Input: part model. Units: mm. Frame: model coordinates. Face numbers are marked on the shaded views. A direction names the side the tool comes from. Round coordinates to 2 decimals unless told otherwise and drop trailing zeros. Loops run counter-clockwise (first coordinate to the right, second up) from the corner with the lowest first, then second, coordinate; pieces in that order, holes last. Notation, with made-up numbers: (37, 5.25) - (81, 5.25) arc R13 ccw to (81, 28.25) - close; hole circle Ø3 at (43, 29). An arc over 180 degrees is marked (long way). One line per question, with ' | ' between items. Start each with the question number.
Item 1: Section C-C, the plane x = 14.5. Return loops of the section in (y, z), plus the area to 3 significant figures.
Item 2: Section A-A, the plane y = 0. Give the number of separate pieces and of enclosed holes in the cut face, plus the area to 3 significant figures.
Item 3: Set-up query: the marked faces 5, 6 and 7. Return all of +Z, -Z, +X, -X, +Y, -Y with unobstructed straight access to the full face (end or side cutting, diameter ignored); none if empty.
Item 4: First-contact query: pin 1 (6.5 mm diameter, centred on x = 8.5, y = 8, fed in from -Z); pin 2 (2 mm diameter, centred on y = -17.5, z = 0.5, fed in from +X); pin 3 (1.8 mm diameter, centred on x = -14.5, z = 3.5, fed in from +Y). Flat tips, straight axial feed; report the tip coordinate or a pass-through.
Item 5: Section D-D, the plane z = 3.25. Return loops of the section in (x, y), plus the area to 3 significant figures.
Item 6: Material intervals for line 1 along Y through (x, z) = (3.5, 1.25); line 2 along X through (y, z) = (0, 1.55); line 3 along Y through (x, z) = (-8, 1), sorted ascending.
Item 7: Draft query along X for the marked faces 1, 2, 3 and 4. Return one class per face: pulls with the +X half, pulls with the -X half, needs draft (parallel to the pull), parting line crosses it, or undercut.
```python
from build123d import *

# Parameters (mm, degrees)
SKETCH_1_R               = 17.4
EXTRUDE_1_DEPTH          = 5.6
SKETCH_2_R               = 1.7
CUT_EXTRUDE_1_DEPTH      = 26.23648153
SKETCH_3_R               = 7
CUT_EXTRUDE_2_DEPTH      = 26.23648153
SKETCH_4_R               = 2.8
CUT_EXTRUDE_3_DEPTH      = 3
SKETCH_5_R               = 1.7
CUT_EXTRUDE_4_DEPTH      = 26.23648153
CUT_EXTRUDE_5_DEPTH      = 2.5
SKETCH_7_W               = 16.1
SKETCH_7_H               = 16.1
CUT_EXTRUDE_6_DEPTH      = 1.5
CHAMFER_1_SIZE           = 0.5
SKETCH_9_W               = 2.2
SKETCH_9_H               = 8
SKETCH_9_W_2             = 8
SKETCH_9_H_2             = 2.2
CUT_EXTRUDE_7_DEPTH      = 26.281613873
BOSS_EXTRUDE1_DEPTH      = 5.6
BOSS_EXTRUDE1_DEPTH_BACK = 4
SKETCH1_R                = 20.65
SKETCH1_R_2              = 17.4
SKETCH3_R                = 23
SKETCH3_R_2              = 20.65
BOSS_EXTRUDE2_DEPTH      = 2.5
SKETCH4_R                = 18
CUT_EXTRUDE3_DEPTH       = 4
SKETCH5_W                = 1
SKETCH5_H                = 8
CUT_EXTRUDE4_DEPTH       = 10
CUT_EXTRUDE6_DEPTH       = 10
FILLET3_R                = 1


with BuildPart() as part:
    # 草图1 → 凸台-拉伸1 (new body)
    with BuildSketch(Plane.XY):
        Circle(SKETCH_1_R)
    extrude(amount=EXTRUDE_1_DEPTH)

    # 草图2 → 切除-拉伸1 (cut, through all)
    with BuildSketch(Plane.XY.offset(5.6)):
        with Locations((-6.717514421, 6.717514421)):
            Circle(SKETCH_2_R)
        with Locations((6.717514421, -6.717514421)):
            Circle(SKETCH_2_R)
    extrude(amount=-CUT_EXTRUDE_1_DEPTH, mode=Mode.SUBTRACT)

    # 草图3 → 切除-拉伸2 (cut, through all)
    with BuildSketch(Plane.XY.offset(5.6)):
        Circle(SKETCH_3_R)
    extrude(amount=-CUT_EXTRUDE_2_DEPTH, mode=Mode.SUBTRACT)

    # 草图4 → 切除-拉伸3 (cut)
    with BuildSketch(Plane.XY.offset(5.6)):
        with Locations((-6.717514421, 6.717514421)):
            Circle(SKETCH_4_R)
        with Locations((6.717514421, -6.717514421)):
            Circle(SKETCH_4_R)
    extrude(amount=-CUT_EXTRUDE_3_DEPTH, mode=Mode.SUBTRACT)

    # 草图5 → 切除-拉伸4 (cut, through all)
    with BuildSketch(Plane.XY.offset(5.6)):
        with Locations((8.05, 8)):
            Circle(SKETCH_5_R)
        with Locations((-8.05, -8)):
            Circle(SKETCH_5_R)
    extrude(amount=-CUT_EXTRUDE_4_DEPTH, mode=Mode.SUBTRACT)

    # 草图6 → 切除-拉伸5 (cut)
    with BuildSketch(Plane(origin=(0, 0, 0), x_dir=(-1, 0, 0), z_dir=(0, 0, -1))):
        Polygon((4.766838493, -8), (6.408419246, -10.84330127), (9.691580754, -10.84330127), (11.333161507, -8), (9.691580754, -5.15669873), (6.408419246, -5.15669873), align=None)
        Polygon((-4.766838493, 8), (-6.408419246, 10.84330127), (-9.691580754, 10.84330127), (-11.333161507, 8), (-9.691580754, 5.15669873), (-6.408419246, 5.15669873), align=None)
    extrude(amount=-CUT_EXTRUDE_5_DEPTH, mode=Mode.SUBTRACT)

    # 草图7 → 切除-拉伸6 (cut)
    with BuildSketch(Plane.XY.offset(5.6)):
        Rectangle(SKETCH_7_W, SKETCH_7_H)
    extrude(amount=-CUT_EXTRUDE_6_DEPTH, mode=Mode.SUBTRACT)

    # 倒角1
    chamfer_1_edges = [part.edges().sort_by_distance(p)[0] for p in [
        (8.05, 1.022551258, 5.6),
        (1.047918985, 8.05, 5.6),
        (-8.05, -1.022551258, 5.6),
        (-1.047918985, -8.05, 5.6),
    ]]
    chamfer(chamfer_1_edges, length=CHAMFER_1_SIZE)

    # 草图8 → 旋转1 (revolve)
    with BuildSketch(Plane(origin=(0, 0, 0), x_dir=(0, 0, -1), z_dir=(1, 0, 0)), mode=Mode.PRIVATE) as revolve_1_sk:
        Polygon((0, 17.4), (0, 17.2), (0.2, 17.4), align=None)
    revolve(revolve_1_sk.sketch.rotate(Axis((0, 0, 0), (0, 0, 1)), 90), axis=Axis((0, 0, 0), (0, 0, 1)))

    # 草图9 → 切除-拉伸7 (cut, through all)
    with BuildSketch(Plane.XY.offset(5.6)):
        with Locations((14.6, 0)):
            Rectangle(SKETCH_9_W, SKETCH_9_H)
        with Locations((0, 14.6)):
            Rectangle(SKETCH_9_W_2, SKETCH_9_H_2)
        with Locations((-14.6, 0)):
            Rectangle(SKETCH_9_W, SKETCH_9_H)
        with Locations((0, -14.6)):
            Rectangle(SKETCH_9_W_2, SKETCH_9_H_2)
    extrude(amount=-CUT_EXTRUDE_7_DEPTH, mode=Mode.SUBTRACT)

    # Sketch1 → Boss-Extrude1 (add, two sides: drawn at the far end of the back side and taken through both)
    with BuildSketch(Plane.XY.offset(-BOSS_EXTRUDE1_DEPTH_BACK)):
        Circle(SKETCH1_R)
        Circle(SKETCH1_R_2, mode=Mode.SUBTRACT)
    extrude(amount=BOSS_EXTRUDE1_DEPTH + BOSS_EXTRUDE1_DEPTH_BACK)

    # Sketch3 → Boss-Extrude2 (add)
    with BuildSketch(Plane(origin=(0, 0, -4), x_dir=(-1, 0, 0), z_dir=(0, 0, -1))):
        Circle(SKETCH3_R)
        with Locations(Location((0, 0, 0), (0, 0, 180))):
            Circle(SKETCH3_R_2, mode=Mode.SUBTRACT)
    extrude(amount=-BOSS_EXTRUDE2_DEPTH)

    # Sketch4 → Cut-Extrude3 (cut)
    with BuildSketch(Plane(origin=(0, 0, -4), x_dir=(-1, 0, 0), z_dir=(0, 0, -1))):
        Circle(SKETCH4_R)
    extrude(amount=-CUT_EXTRUDE3_DEPTH, mode=Mode.SUBTRACT)

    # Sketch5 → Cut-Extrude4 (cut)
    with BuildSketch(Plane(origin=(0, 0, -4), x_dir=(-1, 0, 0), z_dir=(0, 0, -1))):
        with Locations((22.5, 0)):
            Rectangle(SKETCH5_W, SKETCH5_H)
        with Locations((-22.5, 0)):
            Rectangle(SKETCH5_W, SKETCH5_H)
    extrude(amount=-CUT_EXTRUDE4_DEPTH, mode=Mode.SUBTRACT)

    # Sketch7 → Cut-Extrude6 (cut)
    with BuildSketch(Plane(origin=(0, 0, -4), x_dir=(-1, 0, 0), z_dir=(0, 0, -1))):
        with BuildLine():
            Line((0, 18), (0, 22.3))
            Line((0, 22.3), (-2.6, 22.3))
            Line((-2.6, 22.3), (-2.6, 17.811232411))
            ThreePointArc((-2.6, 17.811232411), (-1.303421766, 17.952746077), (0, 18))
        make_face()
        with BuildLine():
            Line((0, 17.5), (0, 18))
            ThreePointArc((0, 18), (-1.303421766, 17.952746077), (-2.6, 17.811232411))
            Line((-2.6, 17.811232411), (-2.6, 17.5))
            Line((-2.6, 17.5), (0, 17.5))
        make_face()
        with BuildLine():
            Line((2.6, 22.3), (0, 22.3))
            Line((0, 22.3), (0, 18))
            ThreePointArc((0, 18), (1.303421766, 17.952746077), (2.6, 17.811232411))
            Line((2.6, 17.811232411), (2.6, 22.3))
        make_face()
        with BuildLine():
            ThreePointArc((2.6, 17.811232411), (1.303421766, 17.952746077), (0, 18))
            Line((0, 18), (0, 17.5))
            Line((0, 17.5), (2.6, 17.5))
            Line((2.6, 17.5), (2.6, 17.811232411))
        make_face()
    extrude(amount=-CUT_EXTRUDE6_DEPTH, mode=Mode.SUBTRACT)

    # Fillet3
    # the kernel refuses this fillet: 1 mm, written as the material it adds along each edge
    with BuildSketch(Plane(origin=(2.6, 22.3, -4), x_dir=(-1, 0, 0), z_dir=(0, 0, 1))) as fillet3_piece_1:
        with BuildLine():
            CenterArc((FILLET3_R, FILLET3_R), FILLET3_R, 180, 90)
            Line((0, FILLET3_R), (-FILLET3_R * 0.02, FILLET3_R))
            Line((-FILLET3_R * 0.02, FILLET3_R), (-FILLET3_R * 0.02, -FILLET3_R * 0.02))
            Line((-FILLET3_R * 0.02, -FILLET3_R * 0.02), (FILLET3_R, -FILLET3_R * 0.02))
            Line((FILLET3_R, -FILLET3_R * 0.02), (FILLET3_R, 0))
        make_face()
    extrude(amount=2.5)
    with BuildSketch(Plane(origin=(-2.6, 22.3, -4), x_dir=(1, 0, 0), z_dir=(0, 0, 1))) as fillet3_piece_2:
        with BuildLine():
            CenterArc((FILLET3_R, -FILLET3_R), FILLET3_R, 90, 90)
            Line((0, -FILLET3_R), (-FILLET3_R * 0.02, -FILLET3_R))
            Line((-FILLET3_R * 0.02, -FILLET3_R), (-FILLET3_R * 0.02, FILLET3_R * 0.02))
            Line((-FILLET3_R * 0.02, FILLET3_R * 0.02), (FILLET3_R, FILLET3_R * 0.02))
            Line((FILLET3_R, FILLET3_R * 0.02), (FILLET3_R, 0))
        make_face()
    extrude(amount=2.5)
    with BuildSketch(Plane(origin=(-2.6, 17.5, -6), x_dir=(0, 1, 0), z_dir=(0, 0, 1))) as fillet3_piece_3_section:
        with BuildLine():
            CenterArc((FILLET3_R, -FILLET3_R), FILLET3_R, 90, 90)
            Line((0, -FILLET3_R), (-FILLET3_R * 0.02, -FILLET3_R))
            Line((-FILLET3_R * 0.02, -FILLET3_R), (-FILLET3_R * 0.02, FILLET3_R * 0.02))
            Line((-FILLET3_R * 0.02, FILLET3_R * 0.02), (FILLET3_R, FILLET3_R * 0.02))
            Line((FILLET3_R, FILLET3_R * 0.02), (FILLET3_R, 0))
        make_face()
    fillet3_piece_3 = extrude(amount=11.6, mode=Mode.PRIVATE)
    fillet3_piece_3 = split(fillet3_piece_3, bisect_by=Plane(origin=(-2.544482942, 18.024809788, 0), z_dir=(0, 0, -1)), keep=Keep.TOP, mode=Mode.PRIVATE)
    fillet3_piece_3 = fillet3_piece_3 - Plane(origin=(0, 0, -2), x_dir=(-1, 0, 0), z_dir=(0, 0, -1)) * Cylinder(18, 28, mode=Mode.PRIVATE)
    fillet3_piece_3 = split(fillet3_piece_3, bisect_by=Plane(origin=(-2.544482942, 18.024809788, -4), z_dir=(0, 0, 1)), keep=Keep.TOP, mode=Mode.PRIVATE)
    add(fillet3_piece_3)
    with BuildSketch(Plane(origin=(-2.6, 17.5, 0), x_dir=(0, 1, 0), z_dir=(0, 0, 1))) as fillet3_piece_4_section:
        with BuildLine():
            CenterArc((FILLET3_R, -FILLET3_R), FILLET3_R, 90, 90)
            Line((0, -FILLET3_R), (-FILLET3_R * 0.02, -FILLET3_R))
            Line((-FILLET3_R * 0.02, -FILLET3_R), (-FILLET3_R * 0.02, FILLET3_R * 0.02))
            Line((-FILLET3_R * 0.02, FILLET3_R * 0.02), (FILLET3_R, FILLET3_R * 0.02))
            Line((FILLET3_R, FILLET3_R * 0.02), (FILLET3_R, 0))
        make_face()
    fillet3_piece_4 = extrude(amount=5.6, mode=Mode.PRIVATE)
    fillet3_piece_4 = fillet3_piece_4 - Plane(origin=(0, 0, 2.8), x_dir=(-1, 0, 0), z_dir=(0, 0, -1)) * Cylinder(18, 16, mode=Mode.PRIVATE)
    add(fillet3_piece_4)
    with BuildSketch(Plane(origin=(-2.6, 17.5, 0), x_dir=(0, 1, 0), z_dir=(0, 0, 1))) as fillet3_piece_5_section:
        with BuildLine():
            CenterArc((FILLET3_R, -FILLET3_R), FILLET3_R, 90, 90)
            Line((0, -FILLET3_R), (-FILLET3_R * 0.02, -FILLET3_R))
            Line((-FILLET3_R * 0.02, -FILLET3_R), (-FILLET3_R * 0.02, FILLET3_R * 0.02))
            Line((-FILLET3_R * 0.02, FILLET3_R * 0.02), (FILLET3_R, FILLET3_R * 0.02))
            Line((FILLET3_R, FILLET3_R * 0.02), (FILLET3_R, 0))
        make_face()
    fillet3_piece_5 = extrude(amount=5.6, mode=Mode.PRIVATE)
    fillet3_piece_5 = fillet3_piece_5 & Plane(origin=(0, 0, 2.8), x_dir=(-1, 0, 0), z_dir=(0, 0, -1)) * Cylinder(18, 16, mode=Mode.PRIVATE)
    add(fillet3_piece_5)
    with BuildSketch(Plane(origin=(2.6, 17.5, -6), x_dir=(-1, 0, 0), z_dir=(0, 0, 1))) as fillet3_piece_6_section:
        with BuildLine():
            CenterArc((FILLET3_R, -FILLET3_R), FILLET3_R, 90, 90)
            Line((0, -FILLET3_R), (-FILLET3_R * 0.02, -FILLET3_R))
            Line((-FILLET3_R * 0.02, -FILLET3_R), (-FILLET3_R * 0.02, FILLET3_R * 0.02))
            Line((-FILLET3_R * 0.02, FILLET3_R * 0.02), (FILLET3_R, FILLET3_R * 0.02))
            Line((FILLET3_R, FILLET3_R * 0.02), (FILLET3_R, 0))
        make_face()
    fillet3_piece_6 = extrude(amount=11.6, mode=Mode.PRIVATE)
    fillet3_piece_6 = split(fillet3_piece_6, bisect_by=Plane(origin=(2.544482942, 18.024809788, 0), z_dir=(0, 0, -1)), keep=Keep.TOP, mode=Mode.PRIVATE)
    fillet3_piece_6 = fillet3_piece_6 - Plane(origin=(0, 0, -2), x_dir=(-1, 0, 0), z_dir=(0, 0, -1)) * Cylinder(18, 28, mode=Mode.PRIVATE)
    fillet3_piece_6 = split(fillet3_piece_6, bisect_by=Plane(origin=(2.544482942, 18.024809788, -4), z_dir=(0, 0, 1)), keep=Keep.TOP, mode=Mode.PRIVATE)
    add(fillet3_piece_6)
    with BuildSketch(Plane(origin=(2.6, 17.5, 0), x_dir=(-1, 0, 0), z_dir=(0, 0, 1))) as fillet3_piece_7_section:
        with BuildLine():
            CenterArc((FILLET3_R, -FILLET3_R), FILLET3_R, 90, 90)
            Line((0, -FILLET3_R), (-FILLET3_R * 0.02, -FILLET3_R))
            Line((-FILLET3_R * 0.02, -FILLET3_R), (-FILLET3_R * 0.02, FILLET3_R * 0.02))
            Line((-FILLET3_R * 0.02, FILLET3_R * 0.02), (FILLET3_R, FILLET3_R * 0.02))
            Line((FILLET3_R, FILLET3_R * 0.02), (FILLET3_R, 0))
        make_face()
    fillet3_piece_7 = extrude(amount=5.6, mode=Mode.PRIVATE)
    fillet3_piece_7 = fillet3_piece_7 & Plane(origin=(0, 0, 2.8), x_dir=(-1, 0, 0), z_dir=(0, 0, -1)) * Cylinder(18, 16, mode=Mode.PRIVATE)
    add(fillet3_piece_7)
    with BuildSketch(Plane(origin=(2.6, 17.5, 0), x_dir=(-1, 0, 0), z_dir=(0, 0, 1))) as fillet3_piece_8_section:
        with BuildLine():
            CenterArc((FILLET3_R, -FILLET3_R), FILLET3_R, 90, 90)
            Line((0, -FILLET3_R), (-FILLET3_R * 0.02, -FILLET3_R))
            Line((-FILLET3_R * 0.02, -FILLET3_R), (-FILLET3_R * 0.02, FILLET3_R * 0.02))
            Line((-FILLET3_R * 0.02, FILLET3_R * 0.02), (FILLET3_R, FILLET3_R * 0.02))
            Line((FILLET3_R, FILLET3_R * 0.02), (FILLET3_R, 0))
        make_face()
    fillet3_piece_8 = extrude(amount=5.6, mode=Mode.PRIVATE)
    fillet3_piece_8 = fillet3_piece_8 - Plane(origin=(0, 0, 2.8), x_dir=(-1, 0, 0), z_dir=(0, 0, -1)) * Cylinder(18, 16, mode=Mode.PRIVATE)
    add(fillet3_piece_8)


solid = part.part
```
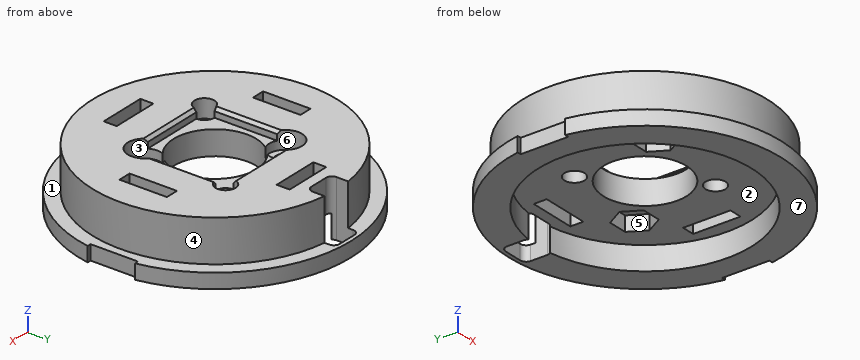
Return value:
1) outline: (-17.85, -4) - (-10.67, -4) - (-10.67, 0) - (-4, 0) - (-4, 5.6) - (-14.7, 5.6) - (-14.7, -1.5) - (-17.85, -1.5) - close; (4, 0) - (10.67, 0) - (10.67, -4) - (17.85, -4) - (17.85, -1.5) - (14.7, -1.5) - (14.7, 5.6) - (4, 5.6) - close | area: 168 mm2
2) separate pieces: 4 | enclosed holes: 0 | area: 153 mm2
3) face 5: -Z | face 6: +Z | face 7: -Z, +X, -X, +Y, -Y
4) pin 1: z = 0 | pin 2: x = 12.42 | pin 3: y = 15.54
5) outline: (-2.6, 18.5) - (-2.6, 20.49) arc R20.65 ccw (long way) to (2.6, 20.49) - (2.6, 18.5) arc R1 cw to (1.6, 17.5) - (-1.6, 17.5) arc R1 cw to start; hole (-15.7, -4) - (-13.5, -4) - (-13.5, 4) - (-15.7, 4) - close; hole circle Ø3.4 at (-8.05, -8); hole (-5.65, 4.13) arc R7 ccw to (4.13, -5.65) arc R2.8 ccw (long way) to (5.65, -4.13) arc R7 ccw to (-4.13, 5.65) arc R2.8 ccw (long way) to start; hole (-4, -15.7) - (4, -15.7) - (4, -13.5) - (-4, -13.5) - close; hole (-4, 13.5) - (4, 13.5) - (4, 15.7) - (-4, 15.7) - close; hole circle Ø3.4 at (8.05, 8); hole (13.5, -4) - (15.7, -4) - (15.7, 4) - (13.5, 4) - close | area: 1,030 mm2
6) line 1: -20.35 to -15.7, -13.5 to -6.06, 6.06 to 13.5, 15.7 to 20.35 | line 2: -20.65 to -15.7, -13.5 to -7, 7 to 13.5, 15.7 to 20.65 | line 3: -19.04 to -10.84, -5.16 to 5.6, 7.83 to 19.04
7) face 1: needs draft | face 2: undercut | face 3: undercut | face 4: parting line crosses it
